The model under review builds one solid part; all positions refer to its coordinate system, in mm. Coordinates: 2 decimals unless noted, no trailing zeros. Loops run counter-clockwise (first coordinate to the right, second up) from the corner with the lowest first, then second, coordinate; pieces in that order, holes last. Notation, with made-up numbers: M 76.25,21.5 L 91.25,21.5 A28 cw 91.25,45.5 Z; hole C -29,0.25 d11. An arc over 180 degrees is marked long. Return JSON: item names as keys, results as strings.
```python
from build123d import *

# Parameters (mm, degrees)
F0_W     = 5
F0_H     = 250
F3_DEPTH = 5.6
F4_DEPTH = 15.001
F5_R     = 2.5
F6_DEPTH = 12.5


with BuildPart() as f1:
    # F0 (on Front) → F1 (revolve)
    with BuildSketch(Plane.XZ):
        with Locations((2.5, 125)):
            Rectangle(F0_W, F0_H)
    revolve(axis=Axis((0, 0, 125), (0, 0, 1)))

    # F2 (on Front) → F3 (join, symmetric)
    with BuildSketch(Plane.XZ):
        Polygon((2.5, 265), (0, 265), (-2.5, 265), (-2.5, 250), (0, 250), (2.5, 250), align=None)
    extrude(amount=F3_DEPTH, both=True)

    # F4 (cut, through all): faces of the model
    f4_faces = [f1.faces().sort_by_distance(p)[0] for p in [
        (0, 5.1676416456, 250),
        (0, -5.1676416456, 250),
    ]]
    extrude(f4_faces, amount=-F4_DEPTH, mode=Mode.SUBTRACT)

    # F5 (on Right) → F6 (cut, symmetric)
    with BuildSketch(Plane.YZ):
        with Locations((0, 261.25)):
            Circle(F5_R)
    extrude(amount=F6_DEPTH, both=True, mode=Mode.SUBTRACT)


solid = f1.part
```
1. To check wall thickness, follow line 1 (Y direction, x = -0.25, z = 261.25); line 2 (Z direction, x = 1.25, y = 0); line 3 (Y direction, x = -2.5, z = 48). State the ranges of each line that lie inside material, in increasing order.
Check values:
{"line 1": "-4.99 to -2.5, 2.5 to 4.99", "line 2": "0 to 258.75, 263.75 to 265", "line 3": "-4.33 to 4.33"}
2. Add section B-B on y = 0. Give the boundary of the cut face in (x, z).
Check values:
{"outline": "M -5,0 L 5,0 L 5,250 L 2.5,250 L 2.5,258.75 L -2.5,258.75 L -2.5,250 L -5,250 Z; M -2.5,263.75 L 2.5,263.75 L 2.5,265 L -2.5,265 Z"}
3. The part is to be moulded in two halves that separate along Z. For faces 1 (the face through (0, 0, 265)), 2 (the face through (0.04, -0.33, 263.73)), 3 (the face through (2.5, 0, 257)), 4 (the face through (0, 0, 0)), say which applies: released by +Z, released by -Z, zero draft, split by the parting line, or undercut.
Check values:
{"face 1": "released by +Z", "face 2": "undercut", "face 3": "zero draft", "face 4": "released by -Z"}
4. Add section A-A on z = 261.25. Give the boundary of the cut face in (x, y), plus the area to 3 significant figures.
Check values:
{"outline": "M -2.5,-4.33 A5 ccw 2.5,-4.33 L 2.5,-2.5 L -2.5,-2.5 Z; M -2.5,2.5 L 2.5,2.5 L 2.5,4.33 A5 ccw -2.5,4.33 Z", "area": "22.8 mm²"}
5. Insertion check: pin 1 Ø1 at (y, z) = (1, 224) entering from +X; pin 2 Ø4.5 at (y, z) = (-1.5, 257.5) entering from -X; pin 3 Ø3 at (x, y) = (3.5, 1) entering from +Z; pin 4 Ø1.5 at (y, z) = (1.5, 90) entering from +X. Each pin has a flat end and moves straight along its axis. Give the tip position at first contact, or say it passes through.
Check values:
{"pin 1": "x = 4.97", "pin 2": "x = -2.5", "pin 3": "z = 265", "pin 4": "x = 4.94"}
6. Add section D-D on z = 105.5. Give the boundary of the cut face in (x, y).
Check values:
{"outline": "C 0,0 d10"}
7. Add section C-C on x = 0.75. Give the boundary of the cut face in (y, z).
Check values:
{"outline": "M -4.94,0 L 4.94,0 L 4.94,265 L -4.94,265 Z; hole C 0,261.25 d5"}
